Job drawing, mm, ordinate dimensions from the low corner. One solid piece. A direction names the side the tool comes from. Round coordinates to 2 decimals unless told otherwise and drop trailing zeros. Order: outer loops, then holes, each group sorted by start corner. A loop starts at its lowest first (then second) coordinate and runs counter-clockwise, first axis right, second up. Notation, with made-up numbers: (-2, 85.5) -> (15, 85.5) arc R21 cw to (15, 113.5) -> close; hole circle Ø3 at (2.25, -5.75). An arc over 180 degrees is marked (long way). Use CSV: the item, a comma, the result in double quotes.
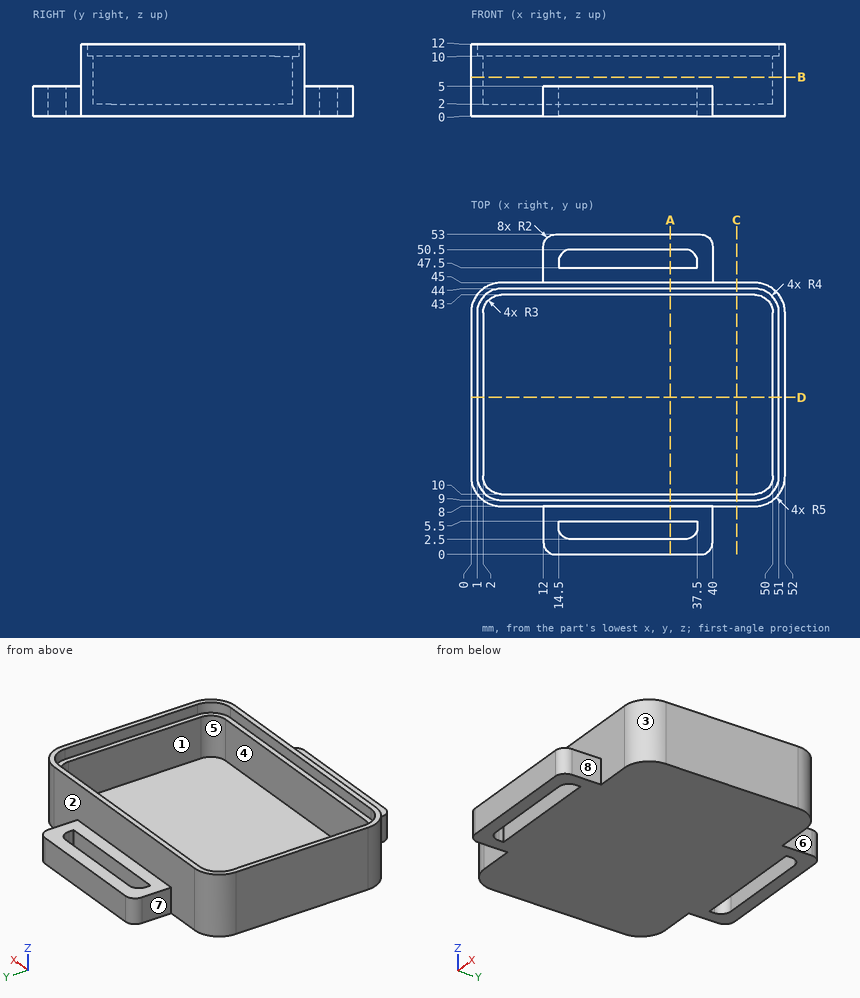
(1) Drop flat-ended pins along their axis: P1, Ø4, axis at x = 41, z = 8, coming from the +Y side; P2, Ø1.5, axis at x = 28.5, z = 2, coming from the -Y side; P3, Ø1, axis at x = 23, z = 11, coming from the -Y side; P4, Ø5.5, axis at y = 4, z = 3, coming from the -X side. Give the stop position or say it passes through.
Reply:
P1,"y = 45"
P2,"y = 0"
P3,"y = 8"
P4,"x = 12"
(2) Cut at C-C, the plane x = 44. Give the cut face in (y, z).
Reply:
outline,"(8, 0) -> (45, 0) -> (45, 12) -> (44, 12) -> (44, 10) -> (43, 10) -> (43, 2) -> (10, 2) -> (10, 10) -> (9, 10) -> (9, 12) -> (8, 12) -> close"
(3) Which spindle directions (+Z, -Z, +X, -X, +Y, -Y) get a long thin tool onto all of the face, cutting with end or side? Do the marked faces 5, 6, 7 and 8. Say none if no direction does.
Reply:
face 5,"+Z"
face 6,"+Z, -Z, +X, +Y"
face 7,"+Z, -Z, -X, +Y"
face 8,"+Z, -Z, +X, -Y"
(4) Probe probe 1 along Y at (x, z) = (46, 10.75); probe 2 along Y at (x, z) = (40, 6.5); probe 3 along Y at (x, z) = (17.5, 4). List the from-to ranges inside material, lowest first. Write a range as [from, to].
Reply:
probe 1,"[8, 9], [44, 45]"
probe 2,"[8, 10], [43, 45]"
probe 3,"[0, 2.5], [5.5, 10], [43, 47.5], [50.5, 53]"
(5) Cut at A-A, the plane x = 33. Give the cut face in (y, z).
Reply:
outline,"(0, 0) -> (2.5, 0) -> (2.5, 5) -> (0, 5) -> close; (5.5, 0) -> (47.5, 0) -> (47.5, 5) -> (45, 5) -> (45, 12) -> (44, 12) -> (44, 10) -> (43, 10) -> (43, 2) -> (10, 2) -> (10, 10) -> (9, 10) -> (9, 12) -> (8, 12) -> (8, 5) -> (5.5, 5) -> close; (50.5, 0) -> (53, 0) -> (53, 5) -> (50.5, 5) -> close"
(6) Pull direction X, two halves, no side cores. Call the marked faces 1, 2, 3 and 4: released by +X, released by -X, zero draft, split by the parting line, or undercut.
Reply:
face 1,"undercut"
face 2,"zero draft"
face 3,"released by +X"
face 4,"undercut"
(7) Cut at D-D, the plane y = 26. Give the cut face in (x, z), then the cut area to 3 significant figures.
Reply:
outline,"(0, 0) -> (52, 0) -> (52, 12) -> (51, 12) -> (51, 10) -> (50, 10) -> (50, 2) -> (2, 2) -> (2, 10) -> (1, 10) -> (1, 12) -> (0, 12) -> close"
area,"140 mm2"
(8) Cut at B-B, the plane z = 6.5. Give the cut face in (x, y).
Reply:
outline,"(0, 13) arc R5 ccw to (5, 8) -> (47, 8) arc R5 ccw to (52, 13) -> (52, 40) arc R5 ccw to (47, 45) -> (5, 45) arc R5 ccw to (0, 40) -> close; hole (2, 13) arc R3 ccw to (5, 10) -> (47, 10) arc R3 ccw to (50, 13) -> (50, 40) arc R3 ccw to (47, 43) -> (5, 43) arc R3 ccw to (2, 40) -> close"
